```python
from build123d import *

# Parameters (mm, degrees)
F1_DEPTH = 25
F2_R     = 16.1752308679


with BuildPart() as f1:
    # F0 (on Top) → F1 (new body)
    with BuildSketch(Plane.XY):
        with BuildLine():
            Line((155.6041836739, 0), (66.094889761, 0))
            ThreePointArc((66.094889761, 0), (58.777489451, -30.2281522154), (38.4455150616, -53.7631548941))
            Line((38.4455150616, -53.7631548941), (155.6041836739, -53.7631548941))
            Line((155.6041836739, -53.7631548941), (155.6041836739, 0))
        make_face()
        with BuildLine():
            ThreePointArc((38.4455150616, -53.7631548941), (58.777489451, -30.2281522154), (66.094889761, 0))
            Line((66.094889761, 0), (0, 0))
            Line((0, 0), (0, -53.7631548941))
            Line((0, -53.7631548941), (38.4455150616, -53.7631548941))
        make_face()
        with BuildLine():
            Line((0, 0), (66.094889761, 0))
            ThreePointArc((66.094889761, 0), (-58.777489451, 30.2281522154), (38.4455150616, -53.7631548941))
            Line((38.4455150616, -53.7631548941), (0, -53.7631548941))
            Line((0, -53.7631548941), (0, 0))
        make_face()
    extrude(amount=F1_DEPTH)

    # F2
    f2_edges = [f1.edges().sort_by_distance(p)[0] for p in [
        (-58.777489, 30.228152, 25),
        (155.604184, -26.881577, 25),
        (110.849537, 0, 25),
        (97.024849, -53.763155, 25),
    ]]
    fillet(f2_edges, radius=F2_R)


solid = f1.part
```
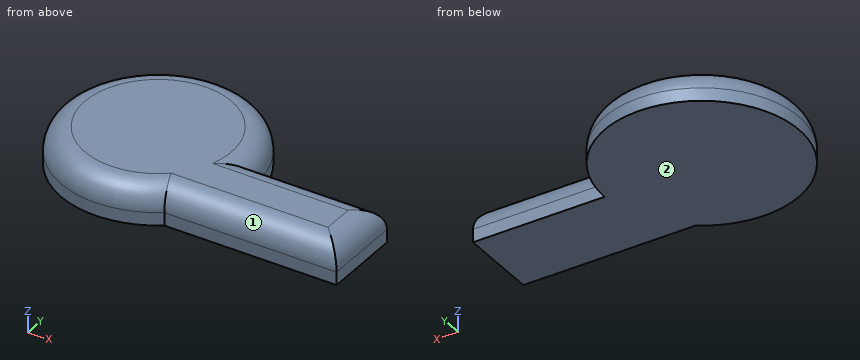
Input: part model. Units: mm. Frame: model coordinates. Face numbers are marked on the shaded views. A direction names the side the tool comes from. Round coordinates to 2 decimals unless told otherwise and drop trailing zeros. Loops run counter-clockwise (first coordinate to the right, second up) from the corner with the lowest first, then second, coordinate; pieces in that order, holes last.
1) Pin query (flat end, axial travel): pin 1 (2.5 mm diameter, centred on x = 128, z = 3.5, fed in from +Y); pin 2 (10 mm diameter, centred on x = 79.5, z = 18, fed in from +Y); pin 3 (5 mm diameter, centred on x = 101.5, y = -9, fed in from +Z). Return the tip coordinate at first contact, or that it passes through.
Ans:
pin 1: stops at y = 0
pin 2: stops at y = -0.55
pin 3: stops at z = 24.31
2) Section query C-C on z = 21.5. Return the cut outline in (x, y), plus the area to 3 significant figures.
Ans:
outline: (36.43, -47.64) - (149.48, -47.64) - (149.48, -6.13) - (59.65, -6.13) arc R59.97 ccw (long way) to start
area: 15,400 mm2
3) Section query A-A on x = 80. Return the cut outline in (y, z), plus the area to 3 significant figures.
Ans:
outline: (-53.76, 0) - (0, 0) - (0, 8.82) arc R16.18 ccw to (-16.18, 25) - (-37.59, 25) arc R16.18 ccw to (-53.76, 8.82) - close
area: 1,230 mm2
4) Material intervals for line 1 (Y direction, x = 113, z = 1.5); line 2 (Y direction, x = -36.5, z = 14.5); line 3 (X direction, y = -32.5, z = 15.25), sorted ascending.
Ans:
line 1: y = -53.76 to 0
line 2: y = -53.86 to 53.86
line 3: x = -56.02 to 154.27
5) Section query B-B on z = 5. Return the cut outline in (x, y), plus the area to 3 significant figures.
Ans:
outline: (38.45, -53.76) - (155.6, -53.76) - (155.6, 0) - (66.09, 0) arc R66.09 ccw (long way) to start
area: 19,000 mm2
6) Set-up query: the marked faces 1 and 2. Return all of +Z, -Z, +X, -X, +Y, -Y with unobstructed straight access to the full face (end or side cutting, diameter ignored); none if empty.
Ans:
face 1: +Z, +X, -Y
face 2: -Z, +X, -X, +Y, -Y
